from build123d import *

# Parameters (mm, degrees)
SKETCH_1_W          = 28
SKETCH_1_H          = 14
EXTRUDE_1_DEPTH     = 22
SKETCH_2_W          = 18
SKETCH_2_H          = 18
CUT_EXTRUDE_1_DEPTH = 22
SKETCH_3_R          = 3.8
CUT_EXTRUDE_2_DEPTH = 29
SKETCH_4_R          = 2
CUT_EXTRUDE_3_DEPTH = 29


with BuildPart() as part:
    # Эскиз1 → Бобышка-Вытянуть1 (new body)
    with BuildSketch(Plane.XY):
        Rectangle(SKETCH_1_W, SKETCH_1_H)
    extrude(amount=EXTRUDE_1_DEPTH)

    # Эскиз2 → Вырез-Вытянуть1 (cut)
    with BuildSketch(Plane.XZ.offset(7)):
        with Locations((0, 13)):
            Rectangle(SKETCH_2_W, SKETCH_2_H)
    extrude(amount=-CUT_EXTRUDE_1_DEPTH, mode=Mode.SUBTRACT)

    # Эскиз3 → Вырез-Вытянуть2 (cut)
    with BuildSketch(Plane(origin=(14, 0, 0), x_dir=(0, 0, -1), z_dir=(1, 0, 0))):
        with Locations((-16.5, 0)):
            Circle(SKETCH_3_R)
    extrude(amount=-CUT_EXTRUDE_2_DEPTH, mode=Mode.SUBTRACT)

    # Эскиз4 → Вырез-Вытянуть3 (cut)
    with BuildSketch(Plane.XY.offset(4)):
        Circle(SKETCH_4_R)
    extrude(amount=-CUT_EXTRUDE_3_DEPTH, mode=Mode.SUBTRACT)


solid = part.part
Source: CAD feature listing. Evaluate the final solid. Frame: model axes, mm. A direction names the side the tool comes from. Give positions to 0.01 mm unless a question says otherwise; leave off trailing zeros. Write each loop counter-clockwise with the first axis right and the second up, starting at its lowest first coordinate (ties: lowest second). Pieces come first, ordered by that corner, then holes. Notation, with made-up numbers: (-39.75, 45.25) -> (-3.75, 45.25) arc R18 ccw to (-3.75, 60.25) -> close; hole circle Ø8 at (33, 28.5). An arc over 180 degrees is marked (long way). Write item = value, one per line.
Q1. Line query: line 1 (Y direction, x = 12, z = 16.5); line 2 (X direction, y = -0.5, z = 12.5); line 3 (Y direction, x = 0, z = 2.15). Output: solid intervals per line, ascending. Write a range as from..to.
Here are the results:
line_1 = -7..-3.8, 3.8..7
line_2 = -14..-9, 9..14
line_3 = -7..-2, 2..7
Q2. Cut plane C-C on y = 0. Return loops of the section in (x, z), then the cut area to 3 significant figures.
Here are the results:
outline = (-14, 0) -> (-2, 0) -> (-2, 4) -> (-9, 4) -> (-9, 12.7) -> (-14, 12.7) -> close; (-14, 20.3) -> (-9, 20.3) -> (-9, 22) -> (-14, 22) -> close; (2, 0) -> (14, 0) -> (14, 12.7) -> (9, 12.7) -> (9, 4) -> (2, 4) -> close; (9, 20.3) -> (14, 20.3) -> (14, 22) -> (9, 22) -> close
area = 200 mm²
Q3. Mould query, pull axis Y, two halves, no side actions, for faces 1 (the face through (-0.2, -7, 3.5)), 2 (the face through (9, 0, 11)), 3 (the face through (-11.465, 0.167, 20.296)). Classes: +Y half, -Y half, draft (parallel to the pull), parting line (faces both ways), or undercut.
Here are the results:
face_1 = -Y half
face_2 = draft
face_3 = undercut
Q4. Cut plane A-A on z = 16.5. Return loops of the section in (x, y).
Here are the results:
outline = (-14, -7) -> (-9, -7) -> (-9, -3.8) -> (-14, -3.8) -> close; (-14, 3.8) -> (-9, 3.8) -> (-9, 7) -> (-14, 7) -> close; (9, -7) -> (14, -7) -> (14, -3.8) -> (9, -3.8) -> close; (9, 3.8) -> (14, 3.8) -> (14, 7) -> (9, 7) -> close
Q5. First-contact query: pin 1 (3 mm diameter, centred on x = -3.5, y = -2, fed in from +Z); pin 2 (10 mm diameter, centred on x = -8.5, z = 13, fed in from -Y). Flat tips, straight axial feed; report the tip coordinate or a pass-through.
Here are the results:
pin_1 = 4
pin_2 = -7
Q6. Cut plane D-D on y = 2.75. Return loops of the section in (x, z).
Here are the results:
outline = (-14, 0) -> (14, 0) -> (14, 13.88) -> (9, 13.88) -> (9, 4) -> (-9, 4) -> (-9, 13.88) -> (-14, 13.88) -> close; (-14, 19.12) -> (-9, 19.12) -> (-9, 22) -> (-14, 22) -> close; (9, 19.12) -> (14, 19.12) -> (14, 22) -> (9, 22) -> close
Q7. Cut plane B-B on x = 0. Return loops of the section in (y, z).
Here are the results:
outline = (-7, 0) -> (-2, 0) -> (-2, 4) -> (-7, 4) -> close; (2, 0) -> (7, 0) -> (7, 4) -> (2, 4) -> close
Q8. Reachability of faces 4 (the face through (-9, 0, 11)), 5 (the face through (14, 0, 11)) from +Z, -Z, +X, -X, +Y, -Y: full face, straight path, thin tool, end or side. Return the list, or none.
Here are the results:
face_4 = +Z, +Y, -Y
face_5 = +Z, -Z, +X, +Y, -Y
